Here's how the part is built. I have some questions about the finished solid (model axes, mm). Face numbers are marked on the shaded views. A direction names the side the tool comes from. Round coordinates to 2 decimals unless told otherwise and drop trailing zeros. Order: outer loops, then holes, each group sorted by start corner. A loop starts at its lowest first (then second) coordinate and runs counter-clockwise, first axis right, second up.
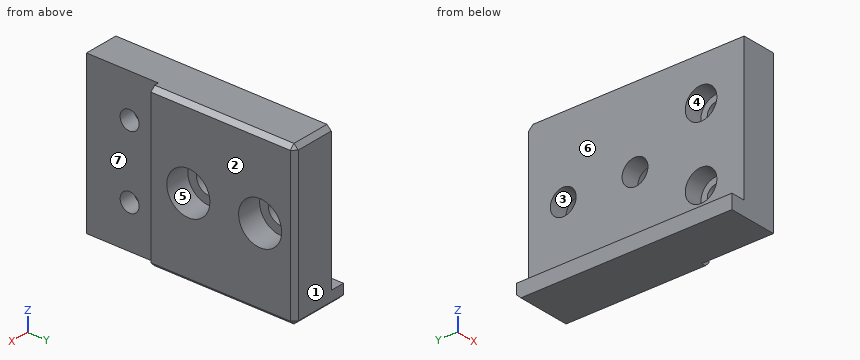
```python
from build123d import *

# Parameters (mm, degrees)
BOSS_EXTRUDE1_DEPTH                                 = 55
SKETCH2_W                                           = 5
SKETCH2_H                                           = 70
BOSS_EXTRUDE2_DEPTH                                 = 5
M5_TAPPED_HOLE1_AT_2_COUNT                          = 2
M5_TAPPED_HOLE1_AT_2_PITCH                          = 20
M5_TAPPED_HOLE1_AT_3_COUNT                          = 2
M5_TAPPED_HOLE1_AT_3_PITCH                          = 40
M5_TAPPED_HOLE1_AT_4_COUNT                          = 2
M5_TAPPED_HOLE1_AT_4_PITCH                          = 60
SKETCH8_W                                           = 104.564197306
SKETCH8_H                                           = 46.562487895
CUT_EXTRUDE1_DEPTH                                  = 87
BOSS_EXTRUDE3_DEPTH                                 = 5
SKETCH10_W                                          = 55
SKETCH10_H                                          = 20
CUT_EXTRUDE2_DEPTH                                  = 3
CBORE_FOR_M6_HEX_SOCKET_HEAD_CAP_SCREW1_D           = 6.6
CBORE_FOR_M6_HEX_SOCKET_HEAD_CAP_SCREW1_CBORE_D     = 11
CBORE_FOR_M6_HEX_SOCKET_HEAD_CAP_SCREW1_CBORE_DEPTH = 6.4
SKETCH13_W                                          = 55
SKETCH13_H                                          = 20
CUT_EXTRUDE3_DEPTH                                  = 5
SKETCH14_W                                          = 5
SKETCH14_H                                          = 55
CUT_EXTRUDE4_DEPTH                                  = 210
SKETCH15_W                                          = 3
SKETCH15_H                                          = 5
CUT_EXTRUDE5_DEPTH                                  = 210
CBORE_FOR_M8_HEX_SOCKET_HEAD_CAP_SCREW1_D           = 9
CBORE_FOR_M8_HEX_SOCKET_HEAD_CAP_SCREW1_CBORE_D     = 15
CBORE_FOR_M8_HEX_SOCKET_HEAD_CAP_SCREW1_CBORE_DEPTH = 8.6
SKETCH18_W                                          = 5
SKETCH18_H                                          = 75
CUT_EXTRUDE6_DEPTH                                  = 210
CHAMFER1_SIZE                                       = 1.5


with BuildPart() as part:
    # Sketch1 → Boss-Extrude1 (new body)
    with BuildSketch(Plane.XY):
        Polygon((0, 0), (110, 0), (110, 20), (20, 20), (20, 70), (0, 70), align=None)
    extrude(amount=BOSS_EXTRUDE1_DEPTH)

    # Sketch2 → Boss-Extrude2 (add)
    with BuildSketch(Plane.ZY):
        with Locations((52.5, 35)):
            Rectangle(SKETCH2_W, SKETCH2_H)
        with Locations((2.5, 35)):
            Rectangle(SKETCH2_W, SKETCH2_H)
    extrude(amount=BOSS_EXTRUDE2_DEPTH)

    # Sketch4 → M5 Tapped Hole1 (revolve, cut)
    with BuildSketch(Plane(origin=(100, 12.5, 55), x_dir=(0, -1, 0), z_dir=(1, 0, 0))):
        Polygon((0, 0), (0, 15.2618073), (2.1, 14), (2.1, 0), align=None)
    m5_tapped_hole1 = revolve(axis=Axis((100, 12.5, 61.35), (0, 0, -1)), mode=Mode.SUBTRACT)

    # M5 Tapped Hole1 at 2: M5 Tapped Hole1 ×2
    with Locations(*[(-i * M5_TAPPED_HOLE1_AT_2_PITCH, 0, 0) for i in range(1, M5_TAPPED_HOLE1_AT_2_COUNT)]):
        add(m5_tapped_hole1, mode=Mode.SUBTRACT)

    # M5 Tapped Hole1 at 3: M5 Tapped Hole1 ×2
    with Locations(*[(-i * M5_TAPPED_HOLE1_AT_3_PITCH, 0, 0) for i in range(1, M5_TAPPED_HOLE1_AT_3_COUNT)]):
        add(m5_tapped_hole1, mode=Mode.SUBTRACT)

    # M5 Tapped Hole1 at 4: M5 Tapped Hole1 ×2
    with Locations(*[(-i * M5_TAPPED_HOLE1_AT_4_PITCH, 0, 0) for i in range(1, M5_TAPPED_HOLE1_AT_4_COUNT)]):
        add(m5_tapped_hole1, mode=Mode.SUBTRACT)

    # Mirror1: M5 Tapped Hole1 across plane
    add(m5_tapped_hole1.mirror(Plane.XY.offset(27.5)), mode=Mode.SUBTRACT)

    # Mirror1 copy 1 sketch → Mirror1 copy 1 (revolve, cut)
    with BuildSketch(Plane(origin=(80, 12.5, 0), x_dir=(0, -1, 0), z_dir=(1, 0, 0))):
        Polygon((0, 0), (0, -15.2618073), (2.1, -14), (2.1, 0), align=None)
    revolve(axis=Axis((80, 12.5, -6.35), (0, 0, -1)), mode=Mode.SUBTRACT)

    # Mirror1 copy 2 sketch → Mirror1 copy 2 (revolve, cut)
    with BuildSketch(Plane(origin=(60, 12.5, 0), x_dir=(0, -1, 0), z_dir=(1, 0, 0))):
        Polygon((0, 0), (0, -15.2618073), (2.1, -14), (2.1, 0), align=None)
    revolve(axis=Axis((60, 12.5, -6.35), (0, 0, -1)), mode=Mode.SUBTRACT)

    # Mirror1 copy 3 sketch → Mirror1 copy 3 (revolve, cut)
    with BuildSketch(Plane(origin=(40, 12.5, 0), x_dir=(0, -1, 0), z_dir=(1, 0, 0))):
        Polygon((0, 0), (0, -15.2618073), (2.1, -14), (2.1, 0), align=None)
    revolve(axis=Axis((40, 12.5, -6.35), (0, 0, -1)), mode=Mode.SUBTRACT)

    # Sketch8 → Cut-Extrude1 (cut)
    with BuildSketch(Plane.XY.offset(55)):
        with Locations((72.282098653, 13.535500523)):
            Rectangle(SKETCH8_W, SKETCH8_H)
    extrude(amount=-CUT_EXTRUDE1_DEPTH, mode=Mode.SUBTRACT)

    # Sketch9 → Boss-Extrude3 (add)
    with BuildSketch(Plane.XZ):
        Polygon((-5, 55), (-5, 50), (0, 50), (0, 5), (-5, 5), (-5, 0), (20, 0), (20, 55), align=None)
    extrude(amount=BOSS_EXTRUDE3_DEPTH)

    # Sketch10 → Cut-Extrude2 (cut)
    with BuildSketch(Plane(origin=(20, 0, 0), x_dir=(0, 0, -1), z_dir=(1, 0, 0))):
        with Locations((-27.5, 10)):
            Rectangle(SKETCH10_W, SKETCH10_H)
    extrude(amount=-CUT_EXTRUDE2_DEPTH, mode=Mode.SUBTRACT)

    # CBORE for M6 Hex Socket Head Cap Screw1 (through all)
    with Locations(Plane.ZY):
        with Locations((15, 10), (40, 10)):
            CounterBoreHole(CBORE_FOR_M6_HEX_SOCKET_HEAD_CAP_SCREW1_D / 2, CBORE_FOR_M6_HEX_SOCKET_HEAD_CAP_SCREW1_CBORE_D / 2, CBORE_FOR_M6_HEX_SOCKET_HEAD_CAP_SCREW1_CBORE_DEPTH)

    # Sketch13 → Cut-Extrude3 (cut)
    with BuildSketch(Plane(origin=(17, 0, 0), x_dir=(0, 0, -1), z_dir=(1, 0, 0))):
        with Locations((-27.5, 10)):
            Rectangle(SKETCH13_W, SKETCH13_H)
    extrude(amount=-CUT_EXTRUDE3_DEPTH, mode=Mode.SUBTRACT)

    # Sketch14 → Cut-Extrude4 (cut)
    with BuildSketch(Plane(origin=(0, 70, 0), x_dir=(1, 0, 0), z_dir=(0, 1, 0))):
        with Locations((17.5, -27.5)):
            Rectangle(SKETCH14_W, SKETCH14_H)
    extrude(amount=-CUT_EXTRUDE4_DEPTH, mode=Mode.SUBTRACT)

    # Sketch15 → Cut-Extrude5 (cut)
    with BuildSketch(Plane.XY.offset(55)):
        with Locations((13.5, -2.5)):
            Rectangle(SKETCH15_W, SKETCH15_H)
    extrude(amount=-CUT_EXTRUDE5_DEPTH, mode=Mode.SUBTRACT)

    # CBORE for M8 Hex Socket Head Cap Screw1 (through all)
    with Locations(Plane(origin=(15, 0, 0), x_dir=(0, 0, -1), z_dir=(1, 0, 0))):
        with Locations((-27.5, 58), (-27.5, 33)):
            CounterBoreHole(CBORE_FOR_M8_HEX_SOCKET_HEAD_CAP_SCREW1_D / 2, CBORE_FOR_M8_HEX_SOCKET_HEAD_CAP_SCREW1_CBORE_D / 2, CBORE_FOR_M8_HEX_SOCKET_HEAD_CAP_SCREW1_CBORE_DEPTH)

    # Sketch18 → Cut-Extrude6 (cut)
    with BuildSketch(Plane(origin=(0, 0, 50), x_dir=(-1, 0, 0), z_dir=(0, 0, -1))):
        with Locations((2.5, 32.5)):
            Rectangle(SKETCH18_W, SKETCH18_H)
    extrude(amount=-CUT_EXTRUDE6_DEPTH, mode=Mode.SUBTRACT)

    # Chamfer1
    chamfer1_edges = [part.edges().sort_by_distance(p)[0] for p in [
        (5, 70, 0),
        (7.5, 70, 55),
        (15, 45, 55),
        (15, 45, 0),
        (15, 70, 27.5),
    ]]
    chamfer(chamfer1_edges, length=CHAMFER1_SIZE)


solid = part.part
```
1. If we section it at B-B, the plane y = 58: Write out the boundary of the cut face in (x, z), and give its area (3 significant figures).
Evaluation:
outline: (-5, 0) - (13.5, 0) - (15, 1.5) - (15, 20) - (6.4, 20) - (6.4, 23) - (0, 23) - (0, 5) - (-5, 5) - close; (0, 32) - (6.4, 32) - (6.4, 35) - (15, 35) - (15, 53.5) - (13.5, 55) - (0, 55) - close
area: 661 mm2
2. If we mould it in two halves opening along Y, with no side actions, what happens to the marked faces 1, 2 and 3? For each: released by +Y, released by -Y, zero draft, split by the parting line, or undercut.
Evaluation:
face 1: released by +Y
face 2: zero draft
face 3: undercut
3. On a 3-axis mill with a long thin cutter (end or side, diameter ignored), from which of +Z, -Z, +X, -X, +Y, -Y can I reach the whole of each face in a straight line? I mean the marked faces 4, 5, 6 and 7. Say none if no direction works.
Evaluation:
face 4: -X
face 5: +X
face 6: +Z, -X, +Y, -Y
face 7: +Z, -Z, +X, -Y
4. If we section it at A-A, the plane z = 40: Write out the boundary of the cut face in (x, y), and give its area (3 significant figures).
Evaluation:
outline: (0, -5) - (12, -5) - (12, 6.7) - (6.4, 6.7) - (6.4, 4.5) - (0, 4.5) - close; (0, 15.5) - (6.4, 15.5) - (6.4, 13.3) - (12, 13.3) - (12, 20) - (15, 20) - (15, 68.5) - (13.5, 70) - (0, 70) - close
area: 942 mm2
5. I need wall thicknesses on probe 1 along Y at (x, z) = (2, 27.5); probe 2 along Z at (x, y) = (7.5, 12); probe 3 along X at (y, z) = (36.5, 16.5). Which ranges of each line are inside material? Lowest first, please.
Evaluation:
probe 1: y = -5 to 28.5, 37.5 to 53.5, 62.5 to 70
probe 2: z = 0 to 12.38, 17.62 to 37.38, 42.62 to 55
probe 3: x = 0 to 15
6. If we section it at D-D, the plane z = 27.5: Write out the boundary of the cut face in (x, y).
Evaluation:
outline: (0, -5) - (12, -5) - (12, 20) - (15, 20) - (15, 25.5) - (6.4, 25.5) - (6.4, 28.5) - (0, 28.5) - close; (0, 37.5) - (6.4, 37.5) - (6.4, 40.5) - (15, 40.5) - (15, 50.5) - (6.4, 50.5) - (6.4, 53.5) - (0, 53.5) - close; (0, 62.5) - (6.4, 62.5) - (6.4, 65.5) - (15, 65.5) - (15, 68.5) - (13.5, 70) - (0, 70) - close
7. I'm going to push flat-ended pins straight in: P1, Ø15, axis at y = 39, z = 39, coming from the -X side; P2, Ø12, axis at y = 57, z = 28, coming from the +X side; P3, Ø20, axis at y = 2, z = 39, coming from the +X side. Where does each tip first touch, or does it pass through?
Evaluation:
P1: stops at x = 0
P2: stops at x = 6.4
P3: stops at x = 12
8. If we section it at C-C, the plane x = 10.5: Write out the boundary of the cut face in (y, z), and give its area (3 significant figures).
Evaluation:
outline: (-5, 0) - (68.5, 0) - (70, 1.5) - (70, 53.5) - (68.5, 55) - (-5, 55) - close; hole circle Ø6.6 at (10, 15); hole circle Ø6.6 at (10, 40); hole circle Ø15 at (33, 27.5); hole circle Ø15 at (58, 27.5)
area: 3,700 mm2
